The listing builds one solid part. Answer for the finished solid, in the listing's coordinates (mm). Round coordinates to 2 decimals unless told otherwise and drop trailing zeros. Write each loop counter-clockwise with the first axis right and the second up, starting at its lowest first coordinate (ties: lowest second). Pieces come first, ordered by that corner, then holes.
Item 1: Find section A-A on y = 5. Give the vertices of the cut face in (x, z), then the cut area to 3 significant figures.
Item 2: Find the intervals of material crossed by probe 1 along X at (y, z) = (8.25, -130); probe 2 along Z at (x, y) = (11.25, 3.5); probe 3 along Y at (x, z) = (10.5, -60.5), in increasing order.
Item 3: This flat-tipped pin is pushed along its axis until it touches: pin 1 (5 mm diameter, centred on x = 2, y = 2.5, fed in from -Z). Where does it stop, or does it pass through?
Item 4: Find section C-C on x = 3.75. Give the vertices of the cut face in (y, z), then the cut area to 3 significant figures.
Item 5: Find section B-B on z = -252. Give the vertices of the cut face in (x, y).
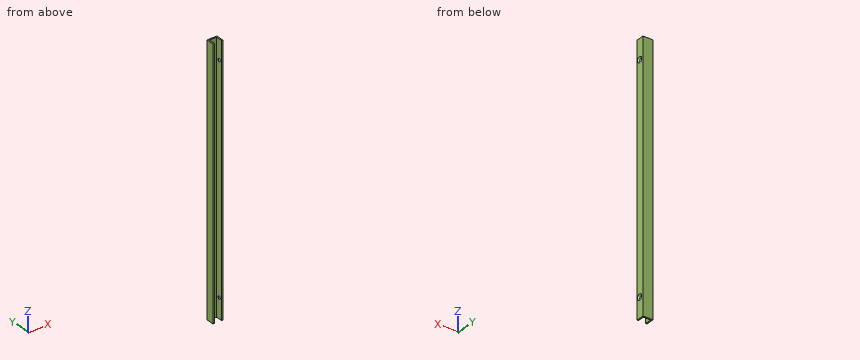
```python
from build123d import *

# Parameters (mm, degrees)
SM_BASE_FLANGE_2_DEPTH = 394
SKETCH_7_R             = 2.3
CUT_EXTRUDE_1_DEPTH    = 2
CHAMFER_1_SIZE         = 2.05


# Sheet-metal steps are written as plain solids
with BuildPart() as part:
    # Эскиз6 → Базовая кромка2 (new body)
    with BuildSketch(Plane.XY):
        Polygon((0, 0), (-2, 0), (-2, 12), (13, 12), (13, 0), (11, 0), (11, 10), (0, 10), align=None)
    extrude(amount=-SM_BASE_FLANGE_2_DEPTH)

    # Эскиз7 → Вырез-Вытянуть1 (cut)
    with BuildSketch(Plane(origin=(13, 0, 0), x_dir=(0, 0, -1), z_dir=(1, 0, 0))):
        with Locations((30, 5)):
            Circle(SKETCH_7_R)
        with Locations((364, 5)):
            Circle(SKETCH_7_R)
    extrude(amount=-CUT_EXTRUDE_1_DEPTH, mode=Mode.SUBTRACT)

    # Фаска1
    # the kernel refuses this chamfer: 2.05 mm, written as the material it takes off along each edge
    with BuildSketch(Plane(origin=(13, 5, -364), x_dir=(0, 0, -1), z_dir=(0, -1, 0))) as chamfer_1_piece_1:
        Polygon((2.3 + CHAMFER_1_SIZE, 0), (2.3, -CHAMFER_1_SIZE), (2.3, 0), align=None)
    revolve(axis=Axis((13, 5, -364), (1, 0, 0)), mode=Mode.SUBTRACT)
    with BuildSketch(Plane(origin=(13, 5, -30), x_dir=(0, 0, -1), z_dir=(0, -1, 0))) as chamfer_1_piece_2:
        Polygon((2.3 + CHAMFER_1_SIZE, 0), (2.3, -CHAMFER_1_SIZE), (2.3, 0), align=None)
    revolve(axis=Axis((13, 5, -30), (1, 0, 0)), mode=Mode.SUBTRACT)


solid = part.part
```
Check values:
1. outline: (-2, -394) - (0, -394) - (0, 0) - (-2, 0) - close; (11, -394) - (13, -394) - (13, -368.35) - (11, -366.35) - close; (11, -361.65) - (13, -359.65) - (13, -34.35) - (11, -32.35) - close; (11, -27.65) - (13, -25.65) - (13, 0) - (11, 0) - close
1. area: 1,550 mm2
2. probe 1: x = -2 to 0, 11 to 13
2. probe 2: z = -394 to -366.12, -361.88 to -32.12, -27.88 to 0
2. probe 3: y = 10 to 12
3. pin 1: stops at z = -394
4. outline: (10, -394) - (12, -394) - (12, 0) - (10, 0) - close
4. area: 788 mm2
5. outline: (-2, 0) - (0, 0) - (0, 10) - (11, 10) - (11, 0) - (13, 0) - (13, 12) - (-2, 12) - close
